from build123d import *

# Parameters (mm, degrees)
SKETCH_1_R      = 1.5
EXTRUDE_1_DEPTH = 2
SKETCH_2_R      = 7
EXTRUDE_2_DEPTH = 2
SKETCH_3_R      = 17.15
EXTRUDE_3_DEPTH = 13.8
FILLET_1_R      = 5
SKETCH_4_R      = 2.5
EXTRUDE_4_DEPTH = 15.1


with BuildPart() as part:
    # 草图1 → 凸台-拉伸1 (new body)
    with BuildSketch(Plane(origin=(0, 0, 0), x_dir=(1, 0, 0), z_dir=(0, 1, 0))):
        with BuildLine():
            ThreePointArc((-2.706611278, 9.702921591), (-10.253048327, 10.253048327), (-9.702921591, 2.706611278))
            ThreePointArc((-9.702921591, 2.706611278), (-8.343447309, 0), (-9.702921591, -2.706611278))
            ThreePointArc((-9.702921591, -2.706611278), (-10.253048327, -10.253048327), (-2.706611278, -9.702921591))
            ThreePointArc((-2.706611278, -9.702921591), (0, -8.343447309), (2.706611278, -9.702921591))
            ThreePointArc((2.706611278, -9.702921591), (10.253048327, -10.253048327), (9.702921591, -2.706611278))
            ThreePointArc((9.702921591, -2.706611278), (8.343447309, 0), (9.702921591, 2.706611278))
            ThreePointArc((9.702921591, 2.706611278), (10.253048327, 10.253048327), (2.706611278, 9.702921591))
            ThreePointArc((2.706611278, 9.702921591), (0, 8.343447309), (-2.706611278, 9.702921591))
        make_face()
        with Locations(Location((-6.717514421, 6.717514421, 0), (0, 0, 270))):
            Circle(SKETCH_1_R, mode=Mode.SUBTRACT)
        with Locations(Location((6.717514421, 6.717514421, 0), (0, 0, 270))):
            Circle(SKETCH_1_R, mode=Mode.SUBTRACT)
        with Locations(Location((6.717514421, -6.717514421, 0), (0, 0, 270))):
            Circle(SKETCH_1_R, mode=Mode.SUBTRACT)
        with Locations(Location((-6.717514421, -6.717514421, 0), (0, 0, 270))):
            Circle(SKETCH_1_R, mode=Mode.SUBTRACT)
    extrude(amount=EXTRUDE_1_DEPTH)

    # 草图2 → 凸台-拉伸2 (add)
    with BuildSketch(Plane(origin=(0, 2, 0), x_dir=(1, 0, 0), z_dir=(0, 1, 0))):
        with Locations(Location((0, 0, 0), (0, 0, 270))):
            Circle(SKETCH_2_R)
    extrude(amount=EXTRUDE_2_DEPTH)

    # 草图3 → 凸台-拉伸3 (add)
    with BuildSketch(Plane(origin=(0, 4, 0), x_dir=(1, 0, 0), z_dir=(0, 1, 0))):
        with Locations(Location((0, 0, 0), (0, 0, 90))):
            Circle(SKETCH_3_R)
    extrude(amount=EXTRUDE_3_DEPTH)

    # 圆角1
    fillet_1_edges = [part.edges().sort_by_distance(p)[0] for p in [
        (0, 17.8, 17.15),
    ]]
    fillet(fillet_1_edges, radius=FILLET_1_R)

    # 草图4 → 凸台-拉伸4 (add)
    with BuildSketch(Plane(origin=(0, 17.8, 0), x_dir=(1, 0, 0), z_dir=(0, 1, 0))):
        with Locations(Location((0, 0, 0), (0, 0, 270))):
            Circle(SKETCH_4_R)
    extrude(amount=EXTRUDE_4_DEPTH)


solid = part.part
Read the model definition and answer for the solid it produces. Units are mm, in the model's axes. A direction names the side the tool comes from. Give positions to 0.01 mm unless a question says otherwise; leave off trailing zeros. Loops run counter-clockwise (first coordinate to the right, second up) from the corner with the lowest first, then second, coordinate; pieces in that order, holes last. Notation, with made-up numbers: (12, 57) -> (68, 57) arc R20 cw to (68, 94) -> close; hole circle Ø3 at (-33, 4). An arc over 180 degrees is marked (long way). Answer as CSV lines item,"result".
Item 1: Find section C-C on y = 25. Give the vertices of the cut face in (x, z).
Returned:
outline,"circle Ø5 at (0, 0)"
Item 2: For faces 5 (the face through (-10.167, 0.986, -10.337)), 6 (the face through (-0.2, 4, -7.4)), 7 (the face through (-8.344, 0.986, -0.044)), 8 (the face through (8.344, 0.986, 0.044)), determine the directions among +Z, -Z, +X, -X, +Y, -Y from which every point of the face is accessible in a straight line to the end or side of a thin tool.
Returned:
face 5,"-Y"
face 6,"none"
face 7,"-X, -Y"
face 8,"+X, -Y"
Item 3: Consider line 1 (Y direction, x = -8, z = 1.5); line 2 (Y direction, x = 3.5, z = -6); line 3 (Y direction, x = -8, z = -6). Determine where each line is inside the solid, lowest interval first. Write a range as [from, to].
Returned:
line 1,"y = [0, 2], [4, 17.8]"
line 2,"y = [0, 17.8]"
line 3,"y = [4, 17.8]"
Item 4: Find section A-A on x = 0. Give the vertices of the cut face in (y, z).
Returned:
outline,"(0, -8.34) -> (2, -8.34) -> (2, -7) -> (4, -7) -> (4, -17.15) -> (12.8, -17.15) arc R5 ccw to (17.8, -12.15) -> (17.8, -2.5) -> (32.9, -2.5) -> (32.9, 2.5) -> (17.8, 2.5) -> (17.8, 12.15) arc R5 ccw to (12.8, 17.15) -> (4, 17.15) -> (4, 7) -> (2, 7) -> (2, 8.34) -> (0, 8.34) -> close"
Item 5: Find section B-B on z = 0. Give the vertices of the cut face in (x, y), plus the area to 3 significant figures.
Returned:
outline,"(-17.15, 4) -> (-7, 4) -> (-7, 2) -> (-8.34, 2) -> (-8.34, 0) -> (8.34, 0) -> (8.34, 2) -> (7, 2) -> (7, 4) -> (17.15, 4) -> (17.15, 12.8) arc R5 ccw to (12.15, 17.8) -> (2.5, 17.8) -> (2.5, 32.9) -> (-2.5, 32.9) -> (-2.5, 17.8) -> (-12.15, 17.8) arc R5 ccw to (-17.15, 12.8) -> close"
area,"599 mm²"
Item 6: Find section D-D on y = 5.5. Give the vertices of the cut face in (x, z).
Returned:
outline,"circle Ø34.3 at (0, 0)"
Item 7: Determine the mould class of faces 1 (the face through (10.167, 0.986, 10.337)), 2 (the face through (-10.337, 0.986, 10.167)), 3 (the face through (0.044, 0.986, -8.344)), 4 (the face through (-6.834, 2.986, -1.517)) for opening direction Z: +Z half, -Z half, draft (parallel to the pull), parting line (faces both ways), or undercut.
Returned:
face 1,"undercut"
face 2,"undercut"
face 3,"-Z half"
face 4,"parting line"
Item 8: Each of these flat-tipped pins is pushed along its axis until it touches: pin 1 (17 mm diameter, centred on x = -7, z = -1.5, fed in from -Y); pin 2 (2 mm diameter, centred on x = 1.5, z = 10, fed in from +Y); pin 3 (3 mm diameter, centred on x = -10.5, y = 11, fed in from +Z); pin 4 (1.8 mm diameter, centred on x = -6.72, z = 6.72, fed in from -Y). Where does it stop, or does it pass through?
Returned:
pin 1,"stops at y = 0"
pin 2,"stops at y = 17.8"
pin 3,"stops at z = 14.6"
pin 4,"stops at y = 4"
